Autodesk Inventor part; units mm, degrees
ref_plane "YZ Plane" through (0, 0, 0) normal (1, 0, 0) x (0, 1, 0)
ref_plane "XZ Plane" through (0, 0, 0) normal (0, 1, 0) x (-1, 0, 0)
ref_plane "XY Plane" through (0, 0, 0) normal (0, 0, 1) x (1, 0, 0)
sketch "Sketch1" plane through (0, 0, 0) normal (0, 1, 0) x (-1, 0, 0)
  line L0 (15.5, 13) -> (-15.5, 13)
  line L1 (-15.5, 13) -> (-15.5, -13)
  line L2 (-15.5, -13) -> (15.5, -13)
  line L3 (15.5, -13) -> (15.5, 13)
  line L4 (15.5, 13) -> (-15.5, -13) construction
  line L5 (-15.5, 13) -> (15.5, -13) construction
  line L6 (18.75, -14.25) -> (-18.75, -14.25)
  line L7 (-18.75, -14.25) -> (-18.75, 14.25)
  line L8 (-18.75, 14.25) -> (18.75, 14.25)
  line L9 (18.75, 14.25) -> (18.75, -14.25)
  line L10 (18.75, -14.25) -> (-18.75, 14.25) construction
  line L11 (-18.75, -14.25) -> (18.75, 14.25) construction
  point P0 (0, 0)
  dimension "d0" = 31
  dimension "d1" = 26
  dimension "d16" = 37.5
  dimension "d17" = 28.5
extrude "Extrusion2" add sketch "Sketch1" along normal blind 1.5 contours L3 L2 L1 L0 | L6 L7 L8 L9
sketch "Sketch2" plane through (0, 1.5, 0) normal (0, 1, 0) x (1, 0, 0)
  line L0 (15.5, 13) -> (-15.5, 13)
  line L1 (-15.5, -13) -> (15.5, -13)
  line L2 (-18.75, -14.25) -> (18.75, -14.25)
  line L3 (18.75, -14.25) -> (18.75, 14.25)
  line L4 (18.75, 14.25) -> (-18.75, 14.25)
  line L5 (-18.75, 14.25) -> (-18.75, -14.25)
  line L6 (15.5, -13) -> (15.5, 13)
  line L7 (-15.5, 13) -> (-15.5, -13)
  point P0 (0, 0)
extrude "Extrusion4" add sketch "Sketch2" along normal blind 1 contours L6 L1 L7 L0
sketch "Sketch3" plane through (0, 2.5, 0) normal (0, 1, 0) x (1, 0, 0)
  circle A0 centre (-14.5, -7) radius 1.5
  circle A1 centre (14.5, -7) radius 1.5
  circle A2 centre (-8.5, 7.75) radius 1.5
  circle A3 centre (8.5, 7.75) radius 1.5
  line L0 (0, -13.0822) -> (0, 13.0822)
  line L1 (-15.5, -13) -> (15.5, -13)
  line L2 (15.5, 13) -> (-15.5, 13)
  line L3 (8, -11.5) -> (-8, -11.5)
  line L4 (-8, -11.5) -> (-8, -2.5)
  line L5 (-8, -2.5) -> (8, -2.5)
  line L6 (8, -2.5) -> (8, -11.5)
  line L7 (8, -11.5) -> (-8, -2.5) construction
  line L8 (-8, -11.5) -> (8, -2.5) construction
  line L9 (4.5, 6) -> (-4.5, 6)
  line L10 (-4.5, 6) -> (-4.5, 9.5)
  line L11 (-4.5, 9.5) -> (4.5, 9.5)
  line L12 (4.5, 9.5) -> (4.5, 6)
  line L13 (4.5, 6) -> (-4.5, 9.5) construction
  line L14 (-4.5, 6) -> (4.5, 9.5) construction
  point P0 (0, 0)
  point P1 (0, -7)
  point P2 (0, 7.75)
  dimension "d25" = 3
  dimension "d26" = 3
  dimension "d27" = 3
  dimension "d28" = 3
  dimension "d29" = 8.5
  dimension "d30" = 8.5
  dimension "d31" = 14.5
  dimension "d32" = 14.5
  dimension "d33" = 6
  dimension "d34" = 6
  dimension "d35" = 5.25
  dimension "d36" = 5.25
  dimension "d37" = 16
  dimension "d38" = 9
  dimension "d39" = 9
  dimension "d40" = 3.5
extrude "Extrusion5" cut sketch "Sketch3" against normal up to surface (2.5 mm away)
sketch "Sketch4" plane through (0, 0, 0) normal (0, -1, 0) x (1, 0, 0)
  line L0 (-15.5, 13) -> (15.5, 13)
  line L1 (15.5, 13) -> (15.5, -13)
  line L2 (-15.5, -13) -> (-15.5, 13)
  line L3 (15.5, -13) -> (-15.5, -13)
  point P0 (0, 0)
sketch "Sketch5" plane through (0, 0, 0) normal (0, -1, 0) x (1, 0, 0)
  line L0 (12, 13.0215) -> (-12, 13.0215)
  line L1 (-12, 13.0215) -> (-12, 1.0215)
  line L2 (-12, 1.0215) -> (12, 1.0215)
  line L3 (12, 1.0215) -> (12, 13.0215)
  line L4 (12, 13.0215) -> (-12, 1.0215) construction
  line L5 (-12, 13.0215) -> (12, 1.0215) construction
  line L6 (6.5, -4.75) -> (-6.5, -4.75)
  line L7 (-6.5, -4.75) -> (-6.5, -10.75)
  line L8 (-6.5, -10.75) -> (6.5, -10.75)
  line L9 (6.5, -10.75) -> (6.5, -4.75)
  line L10 (6.5, -4.75) -> (-6.5, -10.75) construction
  line L11 (-6.5, -4.75) -> (6.5, -10.75) construction
  line L12 (12, 1.0215) -> (6.5, -4.75)
  line L13 (-12, 1.0215) -> (-6.5, -4.75)
  point P0 (0, 0)
  point P1 (0, -7.75)
  point P2 (0, 7.0215)
  dimension "d43" = 24
  dimension "d44" = 12
  dimension "d45" = 13
  dimension "d46" = 6
extrude "Extrusion6" cut sketch "Sketch5" against normal blind 10
equation "\"d30\" = d29"
equation "\"d32\" = d31"
equation "\"d34\" = d33"
equation "\"d36\" = d35"
properties part number "USB outer clamp plate_3DPrint"
The model under review builds one solid part; all positions refer to its coordinate system, in mm. A direction names the side the tool comes from. Coordinates: 2 decimals unless noted, no trailing zeros. Loops run counter-clockwise (first coordinate to the right, second up) from the corner with the lowest first, then second, coordinate; pieces in that order, holes last.
(1) Consider section B-B, the plane y = 1.95. Give the boundary of the cut face in (x, z).
Determined:
outline: (-15.5, -13) - (15.5, -13) - (15.5, 5.88) arc R1.5 cw (long way) to (15.5, 8.12) - (15.5, 13) - (12, 13) - (12, 1.02) - (6.5, -4.75) - (6.5, -10.75) - (-6.5, -10.75) - (-6.5, -4.75) - (-12, 1.02) - (-12, 13) - (-15.5, 13) - (-15.5, 8.12) arc R1.5 cw (long way) to (-15.5, 5.88) - close; hole circle Ø3 at (-8.5, -7.75); hole circle Ø3 at (8.5, -7.75)
(2) Tool access review of faces 1 (the flat face through (0, 2, -13)), 2 (the flat face through (15.5, 2, -3)), 3 (the flat face through (0, 1, 13.022)): name each direction out of +Z, -Z, +X, -X, +Y, -Y from which nothing blocks a thin tool from reaching the whole face with its end or side.
Determined:
face 1: -Z, +X, -X, +Y
face 2: +Z, -Z, +X, +Y
face 3: +Y, -Y
(3) Insertion check: P1, Ø0.5, axis at x = 14, y = 2, coming from the +Z side; P2, Ø0.8, axis at y = 2, z = 10, coming from the -X side; P3, Ø0.8, axis at y = 2, z = 10, coming from the +X side. Each pin has a flat end and moves straight along its axis. Give the tip position at first contact, or say it passes through.
Determined:
P1: stops at z = 13
P2: stops at x = -15.5
P3: stops at x = 15.5
(4) Consider section C-C, the plane z = 7. Give the boundary of the cut face in (x, y), plus the area to 4 significant figures.
Determined:
outline: (-18.75, 0) - (-16, 0) - (-16, 1.5) - (-18.75, 1.5) - close; (-13, 0) - (-12, 0) - (-12, 2.5) - (-13, 2.5) - close; (12, 0) - (13, 0) - (13, 2.5) - (12, 2.5) - close; (16, 0) - (18.75, 0) - (18.75, 1.5) - (16, 1.5) - close
area: 13.25 mm2
(5) Draft analysis for pull direction Z (two halves, no side actions). For faces 4 (the flat face through (0, 1.5, 14)), 5 (the cylindrical face through (-13, 1, 7)), 6 (the flat face through (0, 1, 14.25)), 7 (the flat face through (0, 1, -14.25)), state which applies: +Z half, -Z half, draft (parallel to the pull), parting line (faces both ways), or undercut.
Determined:
face 4: draft
face 5: undercut
face 6: +Z half
face 7: -Z half
(6) Wall thickness on L1, parallel to X at y = 0.7, z = 7; L2, parallel to Z at x = -8.5, y = 1.45; L3, parallel to X at y = 1.05, z = -5: over which ranges is each line inside the solid? List them lowest first.
Determined:
L1: x = -18.75 to -16, -13 to -12, 12 to 13, 16 to 18.75
L2: z = -14.25 to -9.25, -6.25 to -2.65, 13.02 to 14.25
L3: x = -18.75 to -6.5, 6.5 to 18.75
(7) Consider section D-D, the plane z = 12. Give the boundary of the cut face in (x, y), plus the area to 4 significant figures.
Determined:
outline: (-18.75, 0) - (-12, 0) - (-12, 2.5) - (-15.5, 2.5) - (-15.5, 1.5) - (-18.75, 1.5) - close; (12, 0) - (18.75, 0) - (18.75, 1.5) - (15.5, 1.5) - (15.5, 2.5) - (12, 2.5) - close
area: 27.25 mm2
(8) Consider section A-A, the plane x = 6. Give the boundary of the cut face in (y, z).
Determined:
outline: (0, -14.25) - (1.5, -14.25) - (1.5, -13) - (2.5, -13) - (2.5, -10.75) - (0, -10.75) - close; (0, 13.02) - (1.5, 13.02) - (1.5, 14.25) - (0, 14.25) - close
